Work out the finished part from the listing and answer in its coordinate system (mm). Round coordinates to 2 decimals unless told otherwise and drop trailing zeros. Write each loop counter-clockwise with the first axis right and the second up, starting at its lowest first coordinate (ties: lowest second). Pieces come first, ordered by that corner, then holes. Notation, with made-up numbers: M 20.5,79 L 45.5,79 A26 ccw 45.5,117 Z; hole C -9,57.25 d4. An arc over 180 degrees is marked long. Answer in a Markdown table with one row per item.
Autodesk Inventor part; units mm, degrees
ref_plane "YZ Plane" through (0, 0, 0) normal (1, 0, 0) x (0, 1, 0)
ref_plane "XZ Plane" through (0, 0, 0) normal (0, 1, 0) x (-1, 0, 0)
ref_plane "XY Plane" through (0, 0, 0) normal (0, 0, 1) x (1, 0, 0)
sketch "Boceto principal" plane through (0, 0, 0) normal (1, 0, 0) x (0, 1, 0)
  line L0 (0, -1) -> (0, -3)
  line L1 (0, -3) -> (2, -3)
  line L2 (2, -3) -> (2, -2)
  line L3 (2, -2) -> (6, -2)
  line L4 (7, -3) -> (7, -27)
  line L5 (6, -28) -> (2, -28)
  line L6 (2, -28) -> (2, -27)
  line L7 (2, -27) -> (0, -27)
  line L8 (0, -27) -> (0, -29)
  line L9 (1, -30) -> (8, -30)
  line L10 (9, -29) -> (9, -1)
  line L11 (8, 0) -> (1, 0)
  arc A0 (1, 0) -> (0, -1) centre (1, -1) ccw
  arc A1 (7, -3) -> (6, -2) centre (6, -3) ccw
  arc A2 (6, -28) -> (7, -27) centre (6, -27) ccw
  arc A3 (0, -29) -> (1, -30) centre (1, -29) ccw
  arc A4 (8, -30) -> (9, -29) centre (8, -29) ccw
  arc A5 (9, -1) -> (8, 0) centre (8, -1) ccw
extrude "Extrusion1" add sketch "Boceto principal" along normal blind 378
properties part number "Tapa 30x30 378mm" material "PVC, Flexible"
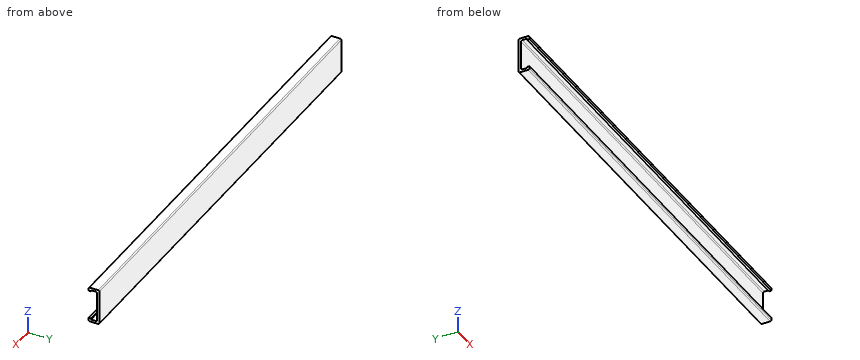
1. The part is cut by section A-A (y = 3.75). Determine the outline of the cut face in (x, z).
Calculated:
| item | result |
|---|---|
| outline | M 0,-30 L 378,-30 L 378,-28 L 0,-28 Z; M 0,-2 L 378,-2 L 378,0 L 0,0 Z |
2. The part is cut by section C-C (z = -6.5). Determine the outline of the cut face in (x, y).
Calculated:
| item | result |
|---|---|
| outline | M 0,7 L 378,7 L 378,9 L 0,9 Z |
3. Consider line 1 along Z through (x, y) = (139.5, 4.5); line 2 along Z through (x, y) = (338, 1.25); line 3 along Y through (x, z) = (120.5, -12.5). Determine where each line is inside the solid, lowest interval first. Write a range as from..to.
Calculated:
| item | result |
|---|---|
| line 1 | z = -30..-28, -2..0 |
| line 2 | z = -30..-27, -3..0 |
| line 3 | y = 7..9 |
4. The part is cut by section B-B (x = 179.5). Determine the outline of the cut face in (y, z).
Calculated:
| item | result |
|---|---|
| outline | M 0,-29 A1 ccw 1,-30 L 8,-30 A1 ccw 9,-29 L 9,-1 A1 ccw 8,0 L 1,0 A1 ccw 0,-1 L 0,-3 L 2,-3 L 2,-2 L 6,-2 A1 cw 7,-3 L 7,-27 A1 cw 6,-28 L 2,-28 L 2,-27 L 0,-27 Z |
5. Given pin 1 (2 mm diameter, centred on x = 86.5, z = -23, fed in from -Y), flat-ended and moving along its own axis, determine where the tip first touches the part or whether it passes through.
Calculated:
| item | result |
|---|---|
| pin 1 | stops at y = 7 |
